```python
from build123d import *

# Parameters (mm, degrees)
SKETCH1_R           = 37
BOSS_EXTRUDE1_DEPTH = 8
FILLET1_R           = 1.5
SKETCH2_R           = 35
CUT_EXTRUDE1_DEPTH  = 53.933921141


with BuildPart() as part:
    # Sketch1 → Boss-Extrude1 (new body)
    with BuildSketch(Plane.YZ):
        with Locations(Location((0, 0, 0), (0, 0, 270))):
            Circle(SKETCH1_R)
    extrude(amount=BOSS_EXTRUDE1_DEPTH)

    # Fillet1
    fillet1_edges = [part.edges().sort_by_distance(p)[0] for p in [
        (0, 0, 37),
        (8, 0, 37),
    ]]
    fillet(fillet1_edges, radius=FILLET1_R)

    # Sketch2 → Cut-Extrude1 (cut, through all)
    with BuildSketch(Plane.YZ.offset(8)):
        with Locations(Location((0, 0, 0), (0, 0, 270))):
            Circle(SKETCH2_R)
    extrude(amount=-CUT_EXTRUDE1_DEPTH, mode=Mode.SUBTRACT)


solid = part.part
```
The listing builds one solid part. Answer for the finished solid, in the listing's coordinates (mm). Coordinates: 2 decimals unless noted, no trailing zeros. Write each loop counter-clockwise with the first axis right and the second up, starting at its lowest first coordinate (ties: lowest second). Pieces come first, ordered by that corner, then holes. Notation, with made-up numbers: (55.25, 7) - (68.25, 7) arc R14 cw to (68.25, 18) - close; hole circle Ø5 at (-13.75, 33.25). An arc over 180 degrees is marked (long way). One line per item, written item: value.
1) Find section A-A (z = 0). Give the vertices of the cut face in (x, y), and give its area (3 significant figures).
Geometry check:
outline: (0, -35.5) arc R1.5 ccw to (1.5, -37) - (6.5, -37) arc R1.5 ccw to (8, -35.5) - (8, -35) - (0, -35) - close; (0, 35) - (8, 35) - (8, 35.5) arc R1.5 ccw to (6.5, 37) - (1.5, 37) arc R1.5 ccw to (0, 35.5) - close
area: 30.1 mm2
2) For a pull along Y with two mould halves and no side action, classify faces 1 (the flat face through (0, -31.4, 15.9)), 2 (the cylindrical face through (4, -21, 28)), 3 (the cylindrical face through (3.96, -14.17, -34.18)) as pulls with the +Y half, pulls with the -Y half, needs draft (parallel to the pull), parting line crosses it, or undercut.
Geometry check:
face 1: needs draft
face 2: undercut
face 3: parting line crosses it
3) Find section B-B (x = 3). Give the vertices of the cut face in (y, z).
Geometry check:
outline: circle Ø74 at (0, 0); hole circle Ø70 at (0, 0)
4) Consider line 1 along Y through (x, z) = (3.25, 0); line 2 along Z through (x, y) = (1.75, -1); line 3 along Z through (x, y) = (2.75, -28.5). Determine where each line is inside the solid, lowest interval first. Write a range as from..to.
Geometry check:
line 1: y = -37..-35, 35..37
line 2: z = -36.99..-34.99, 34.99..36.99
line 3: z = -23.6..-20.32, 20.32..23.6
5) Each of these flat-tipped pins is pushed along its axis until it touches: pin 1 Ø1 at (x, y) = (6.5, 29) entering from -Z; pin 2 Ø4 at (x, y) = (6, -10.5) entering from -Z; pin 3 Ø3 at (x, y) = (4.5, -19.5) entering from -Z. Where does it stop, or does it pass through?
Geometry check:
pin 1: stops at z = -23.6
pin 2: stops at z = -36.01
pin 3: stops at z = -32.33
